```python
from build123d import *

# Parameters (mm, degrees)
F0_W     = 12.7
F0_H     = 50.8
F1_DEPTH = 25.4
F2_W     = 12.7
F2_H     = 12.7
F2_W_2   = 16.51
F2_H_2   = 25.4
F3_DEPTH = 50.801


# Not quite as in the source:
# - a feature names something its author has since deleted; it is built from what else it names


with BuildPart() as f1:
    # F0 (on Front) → F1 (new body, symmetric)
    with BuildSketch(Plane.XZ):
        with Locations((6.35, 25.4)):
            Rectangle(F0_W, F0_H)
        Polygon((12.7, 50.8), (12.7, 0), (25.4, 0), (50.8, 0), (50.8, 25.4), (25.4, 50.8), align=None)
    extrude(amount=F1_DEPTH, both=True)

    # F2 (on face) → F3 (cut, through all)
    with BuildSketch(Plane.XY.offset(50.8)):
        with Locations((6.35, -19.05)):
            Rectangle(F2_W, F2_H)
        with Locations((6.35, 19.05)):
            Rectangle(F2_W, F2_H)
        with Locations((42.545, 0)):
            Rectangle(F2_W_2, F2_H_2)
    extrude(amount=-F3_DEPTH, mode=Mode.SUBTRACT)


solid = f1.part
```
Can you work these out from the model? Positions are in its coordinate system, mm. A direction names the side the tool comes from. Give positions to 0.01 mm unless a question says otherwise; leave off trailing zeros. Order: outer loops, then holes, each group sorted by start corner. A loop starts at its lowest first (then second) coordinate and runs counter-clockwise, first axis right, second up. Notation, with made-up numbers: M 60.5,-39 L 88.5,-39 A14 cw 88.5,-33 Z; hole C 26.5,33 d4. An arc over 180 degrees is marked long. One line per item, written item: value.
1) I want a section at C-C, the plane y = 19. List the corners of the cut face in (x, z) for me, plus the area to 3 significant figures.
Answer sheet:
outline: M 12.7,0 L 50.8,0 L 50.8,25.4 L 25.4,50.8 L 12.7,50.8 Z
area: 1,610 mm^2
2) I want a section at A-A, the plane x = 36. List the corners of the cut face in (y, z) for me, plus the area to 3 significant figures.
Answer sheet:
outline: M -25.4,0 L -12.7,0 L -12.7,40.2 L -25.4,40.2 Z; M 12.7,0 L 25.4,0 L 25.4,40.2 L 12.7,40.2 Z
area: 1,020 mm^2
3) On a 3-axis mill with a long thin cutter (end or side, diameter ignored), from which of +Z, -Z, +X, -X, +Y, -Y can I reach the whole of each face in a straight line? I mean faces 1 (the face through (6, -12.7, 26)), 2 (the face through (50.8, -19, 13)), 3 (the face through (42, -12.7, 17)), 4 (the face through (12.7, 19, 26)). Say none if no direction works.
Answer sheet:
face 1: +Z, -Z, -X, -Y
face 2: +Z, -Z, +X, +Y, -Y
face 3: +Z, -Z, +X
face 4: +Z, -Z, -X, +Y
4) We'd pull the mould along Y, two halves only. Please class faces 5 (the face through (42, 12.7, 17)), 6 (the face through (31, 25.4, 20)), 7 (the face through (16, 0, 50.8)): released by +Y, released by -Y, zero draft, split by the parting line, or undercut.
Answer sheet:
face 5: undercut
face 6: released by +Y
face 7: zero draft
5) Please list where these lines run through material, in increasing order: line 1 along Y through (x, z) = (36.5, 37.5); line 2 along Y through (x, z) = (6, 29.5); line 3 along X through (y, z) = (0.5, 9.5).
Answer sheet:
line 1: y = -25.4 to -12.7, 12.7 to 25.4
line 2: y = -12.7 to 12.7
line 3: x = 0 to 34.29
6) For P1, Ø4, axis at y = 20, z = 18, coming from the -X side; P2, Ø14, axis at x = 7.5, z = 37.5, coming from the +Y side; P3, Ø4, axis at x = 7, z = 30, coming from the -Y side; P4, Ø12.5, axis at y = 1, z = 24, coming from the +X side, each with a flat end and sliding along its axis, tell me the tip position at first contact or that it passes through.
Answer sheet:
P1: stops at x = 12.7
P2: stops at y = 25.4
P3: stops at y = -12.7
P4: stops at x = 34.29
7) I want a section at B-B, the plane z = 45. List the corners of the cut face in (x, y) for me.
Answer sheet:
outline: M 0,-12.7 L 12.7,-12.7 L 12.7,-25.4 L 31.2,-25.4 L 31.2,25.4 L 12.7,25.4 L 12.7,12.7 L 0,12.7 Z
8) I want a section at D-D, the plane x = 45.5. List the corners of the cut face in (y, z) for me.
Answer sheet:
outline: M -25.4,0 L -12.7,0 L -12.7,30.7 L -25.4,30.7 Z; M 12.7,0 L 25.4,0 L 25.4,30.7 L 12.7,30.7 Z
